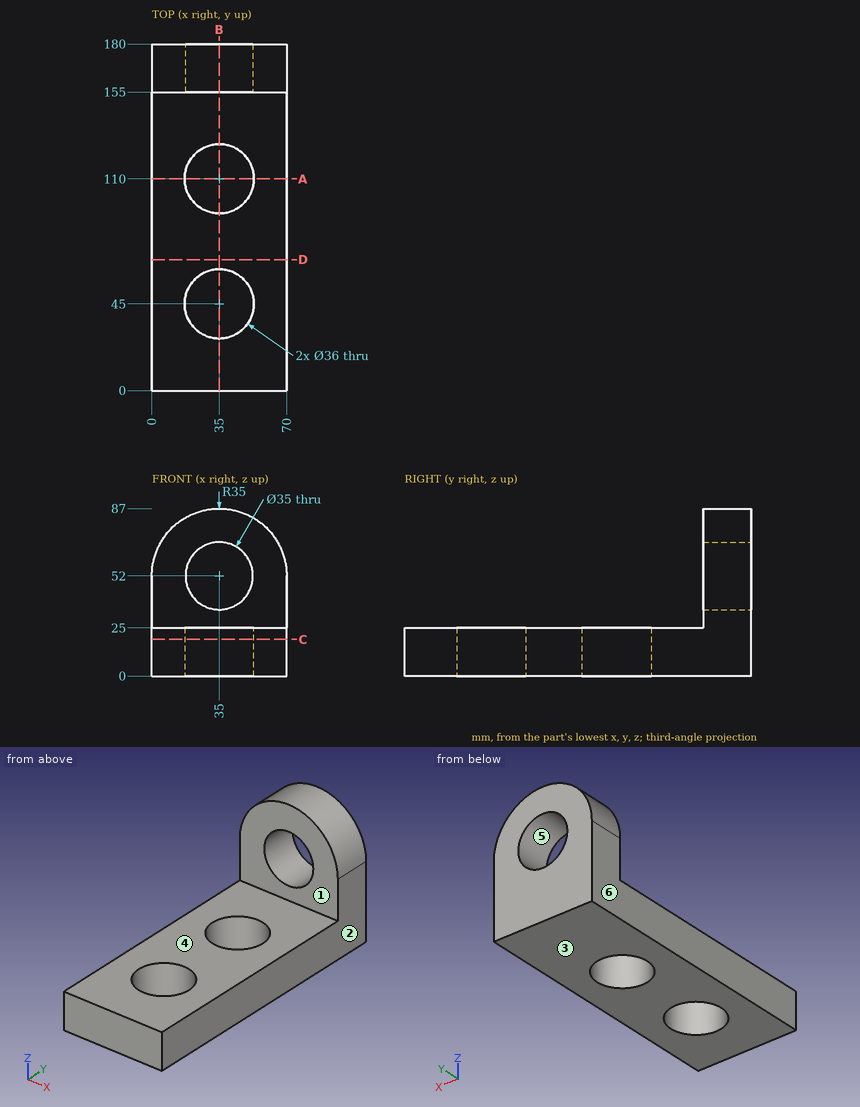
Can you work these out from the drawing? Everything is in mm from the part's minimum corner. A direction names the side the tool comes from. Give positions to 0.01 mm unless a question says otherwise; leave off trailing zeros. Order: outer loops, then holes, each group sorted by start corner. A loop starts at its lowest first (then second) coordinate and runs counter-clockwise, first axis right, second up. Notation, with made-up numbers: M 41,-23.5 L 47,-23.5 A31 cw 47,7.5 Z; hole C 35,-22.5 d5. An arc over 180 degrees is marked long. Use a Markdown table: item, result. Add a question column.
1. On a 3-axis mill with a long thin cutter (end or side, diameter ignored), from which of +Z, -Z, +X, -X, +Y, -Y can I reach the whole of each face in a straight line? I mean the marked faces 1 and 2. Say none if no direction works.
2. Suppose I cut it at B-B (x = 35). List the corners of the cut face in (y, z) for me, and give its area (4 significant figures).
3. I need wall thicknesses on probe 1 along Y at (x, z) = (35, 12); probe 2 along Z at (x, y) = (35, 175.25); probe 3 along X at (y, z) = (110, 18). Which ranges of each line are inside material? Lowest first, please. Write a range as from..to.
4. Suppose I cut it at C-C (z = 19). List the corners of the cut face in (x, y) for me, and give its area (3 significant figures).
5. Suppose I cut it at A-A (y = 110). List the corners of the cut face in (x, z) for me.
6. If we mould it in two halves opening along Z, with no side actions, what happens to the marked faces 3, 4, 5 and 6? For each: +Z half, -Z half, draft (parallel to the pull), parting line (faces both ways), or undercut.
7. For pin 1 Ø1.5 at (x, z) = (42, 35.5) entering from -Y, with a flat end and sliding along its axis, tell me the tip position at first contact or that it passes through.
8. Suppose I cut it at D-D (y = 68). List the corners of the cut face in (x, z) for me.
Results list:
| question | item | result |
|---|---|---|
| 1 | face 1 | +Z, +X, -X, -Y |
| 1 | face 2 | +Z, -Z, +X, +Y, -Y |
| 2 | outline | M 0,0 L 27,0 L 27,25 L 0,25 Z; M 63,0 L 92,0 L 92,25 L 63,25 Z; M 128,0 L 180,0 L 180,34.5 L 155,34.5 L 155,25 L 128,25 Z; M 155,69.5 L 180,69.5 L 180,87 L 155,87 Z |
| 2 | area | 3,375 mm² |
| 3 | probe 1 | y = 0..27, 63..92, 128..180 |
| 3 | probe 2 | z = 0..34.5, 69.5..87 |
| 3 | probe 3 | x = 0..17, 53..70 |
| 4 | outline | M 0,0 L 70,0 L 70,180 L 0,180 Z; hole C 35,45 d36; hole C 35,110 d36 |
| 4 | area | 10,600 mm² |
| 5 | outline | M 0,0 L 17,0 L 17,25 L 0,25 Z; M 53,0 L 70,0 L 70,25 L 53,25 Z |
| 6 | face 3 | -Z half |
| 6 | face 4 | +Z half |
| 6 | face 5 | undercut |
| 6 | face 6 | draft |
| 7 | pin 1 | stops at y = 155 |
| 8 | outline | M 0,0 L 70,0 L 70,25 L 0,25 Z |
